Answer from the drawing. Dimensions are ordinates in mm from the lowest x, y and z of the part. Coordinates: 2 decimals unless noted, no trailing zeros. Write each loop counter-clockwise with the first axis right and the second up, starting at its lowest first coordinate (ties: lowest second). Pieces come first, ordered by that corner, then holes.
(1) Section A-A on z = 74 is taken. Write down the section's boundary in (x, y).
(2) Section B-B on x = 93 is taken. Write down the section's boundary in (y, z), then the cut area to 3 significant figures.
(3) Section C-C on z = 207 is taken. Write down the section's boundary in (x, y), then the cut area to 3 significant figures.
(4) Find the intervals of material crossed by probe 1 along Z at (x, y) = (107.5, 2.65); probe 2 along X at (y, z) = (1.1, 196); probe 3 along X at (y, z) = (2.1, 119), in increasing order.
(5) Section D-D on y = 1.25 is taken. Write down the section's boundary in (x, z), then the cut area to 3 significant figures.
(6) Given pin 1 (1 mm diameter, centred on x = 213.5, y = 2, fed in from +Z), flat-ended and moving along its own axis, determine where the tip first touches the part or whether it passes through.
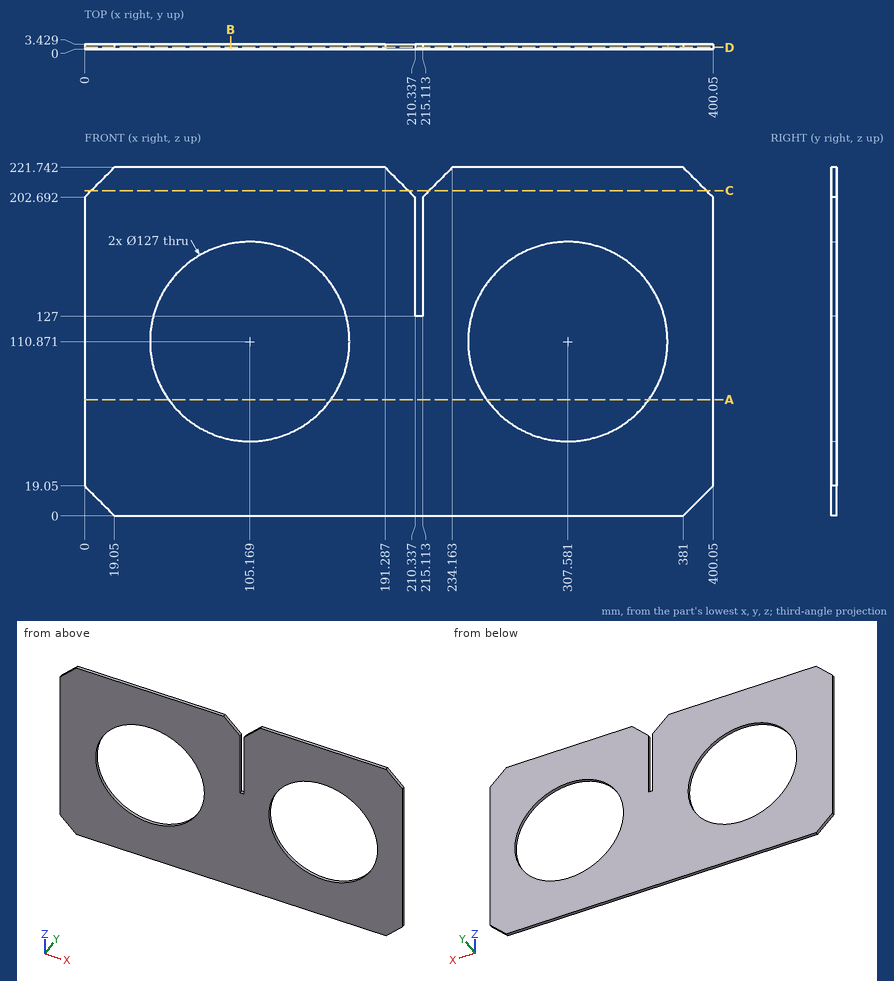
Response:
1. outline: (0, 0) - (53.47, 0) - (53.47, 3.43) - (0, 3.43) - close; (156.87, 0) - (255.88, 0) - (255.88, 3.43) - (156.87, 3.43) - close; (359.28, 0) - (400.05, 0) - (400.05, 3.43) - (359.28, 3.43) - close
2. outline: (0, 0) - (3.43, 0) - (3.43, 48.55) - (0, 48.55) - close; (0, 173.19) - (3.43, 173.19) - (3.43, 221.74) - (0, 221.74) - close
2. area: 333 mm2
3. outline: (4.31, 0) - (206.03, 0) - (206.03, 3.43) - (4.31, 3.43) - close; (219.42, 0) - (395.74, 0) - (395.74, 3.43) - (219.42, 3.43) - close
3. area: 1,300 mm2
4. probe 1: z = 0 to 47.41, 174.33 to 221.74
4. probe 2: x = 0 to 210.34, 215.11 to 400.05
4. probe 3: x = 0 to 42.19, 168.15 to 244.6, 370.56 to 400.05
5. outline: (0, 19.05) - (19.05, 0) - (381, 0) - (400.05, 19.05) - (400.05, 202.69) - (381, 221.74) - (234.16, 221.74) - (215.11, 202.69) - (215.11, 127) - (210.34, 127) - (210.34, 202.69) - (191.29, 221.74) - (19.05, 221.74) - (0, 202.69) - close; hole circle Ø127 at (105.17, 110.87); hole circle Ø127 at (307.58, 110.87)
5. area: 61,800 mm2
6. pin 1: stops at z = 127
